The model under review builds one solid part; all positions refer to its coordinate system, in mm. Face numbers are marked on the shaded views. A direction names the side the tool comes from. Round coordinates to 2 decimals unless told otherwise and drop trailing zeros. Order: outer loops, then holes, each group sorted by start corner. A loop starts at its lowest first (then second) coordinate and runs counter-clockwise, first axis right, second up. Notation, with made-up numbers: M 89,8 L 109,8 A23 ccw 109,29 Z; hole C 53.5,-25.5 d4. An arc over 180 degrees is marked long. Answer as a JSON object with one key per item and string values. Group by question number.
1) Consider section D-D, the plane z = -25. Write out the cut boundary in (x, y), then the cut area to 3 significant figures.
2) Insertion check: pin 1 Ø10 at (x, y) = (-5.5, 7.5) entering from +Z; pin 2 Ø1.9 at (x, y) = (0, 14) entering from +Z; pin 3 Ø6 at (x, z) = (14, -27.5) entering from -Y. Each pin has a flat end and moves straight along its axis. Give the tip position at first contact, or say it passes through.
3) For the marked faces 1 and 2, list the 3-axis set-ups (+Z, -Z, +X, -X, +Y, -Y) from which the entire face can be reached by the end or side of a thin tool; tool diameter is ignored.
4) Consider section B-B, the plane z = -1. Write out the cut boundary in (x, y).
5) To check wall thickness, follow line 1 (Y direction, x = 0, z = -1.75); line 2 (Z direction, x = -0.5, y = 13); line 3 (Z direction, x = 8, y = 0). State the ranges of each line that lie inside material, in increasing order.
6) Consider section C-C, the plane x = -8.5. Write out the cut boundary in (y, z).
7) Consider section A-A, the plane y = 0. Write out the cut boundary in (x, z).
```python
from build123d import *

# Parameters (mm, degrees)
SKETCH1_R           = 19
BOSS_EXTRUDE1_DEPTH = 35.5
SKETCH2_R           = 10
BOSS_EXTRUDE2_DEPTH = 5
SKETCH3_R           = 3
BOSS_EXTRUDE3_DEPTH = 13
SKETCH4_R           = 1.174286688
CUT_EXTRUDE1_DEPTH  = 5
CIRPATTERN1_COUNT   = 6


with BuildPart() as part:
    # Sketch1 → Boss-Extrude1 (new body)
    with BuildSketch(Plane.XY):
        Circle(SKETCH1_R)
    extrude(amount=-BOSS_EXTRUDE1_DEPTH)

    # Sketch2 → Boss-Extrude2 (add)
    with BuildSketch(Plane.XY):
        Circle(SKETCH2_R)
    extrude(amount=BOSS_EXTRUDE2_DEPTH)

    # Sketch3 → Boss-Extrude3 (add)
    with BuildSketch(Plane.XY.offset(5)):
        Circle(SKETCH3_R)
    extrude(amount=BOSS_EXTRUDE3_DEPTH)

    # Sketch4 → Cut-Extrude1 (cut)
    with BuildSketch(Plane.XY):
        with Locations((0, 14)):
            Circle(SKETCH4_R)
    cut_extrude1 = extrude(amount=-CUT_EXTRUDE1_DEPTH, mode=Mode.SUBTRACT)

    # CirPattern1: Cut-Extrude1 ×6 about axis
    cirpattern1_axis = Axis((0, 0, 0), (0, 0, 1))
    for i in range(1, CIRPATTERN1_COUNT):
        add(cut_extrude1.rotate(cirpattern1_axis, i * 360 / CIRPATTERN1_COUNT), mode=Mode.SUBTRACT)


solid = part.part
```
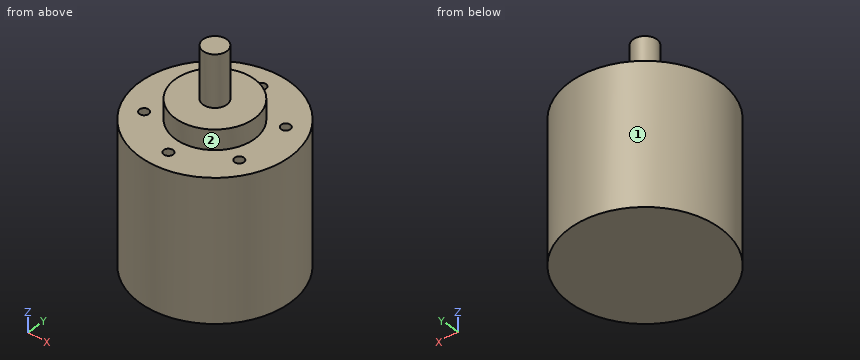
Results list:
{
 "1": {"outline": "C 0,0 d38", "area": "1,130 mm^2"},
 "2": {"pin 1": "z = 5", "pin 2": "z = -5", "pin 3": "y = -15.49"},
 "3": {"face 1": "+Z, -Z", "face 2": "+Z"},
 "4": {"outline": "C 0,0 d38; hole C -12.12,-7 d2.35; hole C -12.12,7 d2.35; hole C 0,-14 d2.35; hole C 0,14 d2.35; hole C 12.12,-7 d2.35; hole C 12.12,7 d2.35"},
 "5": {"line 1": "-19 to -15.17, -12.83 to 12.83, 15.17 to 19", "line 2": "-35.5 to -5", "line 3": "-35.5 to 5"},
 "6": {"outline": "M -16.99,-35.5 L 16.99,-35.5 L 16.99,0 L 5.27,0 L 5.27,5 L -5.27,5 L -5.27,0 L -16.99,0 Z"},
 "7": {"outline": "M -19,-35.5 L 19,-35.5 L 19,0 L 10,0 L 10,5 L 3,5 L 3,18 L -3,18 L -3,5 L -10,5 L -10,0 L -19,0 Z"}
}
